from build123d import *

# Parameters (mm, degrees)
SKETCH_1_W      = 8
SKETCH_1_H      = 3
SKETCH_1_R      = 1.6
EXTRUDE_1_DEPTH = 3


with BuildPart() as part:
    # 草图1 → 凸台-拉伸1 (new body)
    with BuildSketch(Plane.XY):
        Polygon((0, 140), (0, 146), (4, 146), (4, 162), (0, 162), (-44, 162), (-44, 38), (4, 38), (4, 54), (0, 54), (0, 74), (-5, 74), (-5, 94), (4, 94), (4, 114), (0, 114), (0, 120), (-5, 120), (-5, 118), (-8, 118), (-8, 120), (-12, 120), (-12, 124), (-8, 124), (-8, 126), (-5, 126), (-5, 124), (0, 124), (0, 136), (-5, 136), (-5, 134), (-8, 134), (-8, 136), (-12, 136), (-12, 140), (-8, 140), (-8, 142), (-5, 142), (-5, 140), align=None)
        with Locations((-12, 54.5)):
            Rectangle(SKETCH_1_W, SKETCH_1_H, mode=Mode.SUBTRACT)
        with Locations((2, 46)):
            Circle(SKETCH_1_R, mode=Mode.SUBTRACT)
        Polygon((-39, 130), (-32, 130), (-29, 130), (-29, 127), (-39, 127), align=None, mode=Mode.SUBTRACT)
        with Locations((2, 154)):
            Circle(SKETCH_1_R, mode=Mode.SUBTRACT)
    extrude(amount=EXTRUDE_1_DEPTH)


solid = part.part
Geometry: final body of the model. Coordinates: model frame, mm. A direction names the side the tool comes from. Give positions to 0.01 mm unless a question says otherwise; leave off trailing zeros. Order: outer loops, then holes, each group sorted by start corner. A loop starts at its lowest first (then second) coordinate and runs counter-clockwise, first axis right, second up. Notation, with made-up numbers: (-31.75, 75) - (-27.75, 75) arc R9 cw to (-27.75, 81) - close; hole circle Ø9 at (29.25, 58). An arc over 180 degrees is marked (long way). Use CSV: the item, a comma, the result in double quotes.
1. Section query C-C (x = -33). Output: boundary loops of the cut face in (y, z).
Answers below:
outline,"(38, 0) - (127, 0) - (127, 3) - (38, 3) - close; (130, 0) - (162, 0) - (162, 3) - (130, 3) - close"
2. Section query B-B (y = 46). Output: boundary loops of the cut face in (x, z).
Answers below:
outline,"(-44, 0) - (0.4, 0) - (0.4, 3) - (-44, 3) - close; (3.6, 0) - (4, 0) - (4, 3) - (3.6, 3) - close"
3. Mould query, pull axis Y, two halves, no side actions, for faces 4 (the face through (-8, 135, 1)), 5 (the face through (-44, 101, 1)). Classes: +Y half, -Y half, draft (parallel to the pull), parting line (faces both ways), or undercut.
Answers below:
face 4,"undercut"
face 5,"draft"
4. Material intervals for line 1 along Y through (x, z) = (2, 2.15); line 2 along Y through (x, z) = (-3, 2.8); line 3 along Y through (x, z) = (-7, 0.55), sorted ascending. Write a range as from..to.
Answers below:
line 1,"38..44.4, 47.6..54, 94..114, 146..152.4, 155.6..162"
line 2,"38..74, 94..120, 124..136, 140..162"
line 3,"38..118, 126..134, 142..162"
5. Section query D-D (y = 90). Output: boundary loops of the cut face in (x, z).
Answers below:
outline,"(-44, 0) - (-5, 0) - (-5, 3) - (-44, 3) - close"
6. Access query for faces 1 (the face through (0, 143, 1)), 2 (the face through (-12, 56, 1)), 3 (the face through (4, 104, 1)). Directions: +Z, -Z, +X, -X, +Y, -Y. A direction counts if a zero-diameter tool reaches every point of the face in a straight line with its end or side. Return the directions, or none.
Answers below:
face 1,"+Z, -Z, +X"
face 2,"+Z, -Z"
face 3,"+Z, -Z, +X, +Y, -Y"
7. Section query A-A (x = 2). Output: boundary loops of the cut face in (y, z).
Answers below:
outline,"(38, 0) - (44.4, 0) - (44.4, 3) - (38, 3) - close; (47.6, 0) - (54, 0) - (54, 3) - (47.6, 3) - close; (94, 0) - (114, 0) - (114, 3) - (94, 3) - close; (146, 0) - (152.4, 0) - (152.4, 3) - (146, 3) - close; (155.6, 0) - (162, 0) - (162, 3) - (155.6, 3) - close"
8. Contact query for flat-ended pins moving along their axis: pin 1 (1.5 mm diameter, centred on y = 88, z = 1, fed in from +X); pin 2 (12 mm diameter, centred on x = -34, y = 89, fed in from -Z); pin 3 (1.5 mm diameter, centred on y = 121.5, z = 1.5, fed in from +X); pin 4 (0.6 mm diameter, centred on y = 125, z = 1.5, fed in from +X). Output: stop coordinate, or through.
Answers below:
pin 1,"x = -5"
pin 2,"z = 0"
pin 3,"x = -12"
pin 4,"x = 0"
